The model under review builds one solid part; all positions refer to its coordinate system, in mm. Face numbers are marked on the shaded views. A direction names the side the tool comes from. Round coordinates to 2 decimals unless told otherwise and drop trailing zeros. Write each loop counter-clockwise with the first axis right and the second up, starting at its lowest first coordinate (ties: lowest second). Pieces come first, ordered by that corner, then holes.
Item 1: Add section D-D (y = 12.5). Give the boundary of the cut face in (x, z).
Item 2: Add section C-C (x = -3). Give the boundary of the cut face in (y, z), plus the area to 3 significant figures.
Item 3: Add section A-A (z = -0.5). Give the boundary of the cut face in (x, y), plus the area to 3 significant figures.
Item 4: Clearance check with flat-ended pins moving along their axes: pin 1 Ø2 at (x, z) = (17, -1) entering from +Y; pin 2 Ø4 at (x, z) = (0, 15.5) entering from -Y; pin 3 Ø4 at (y, z) = (49, -12.5) entering from +X; pin 4 Ø0.9 at (x, z) = (16.5, -0.5) entering from -Y. State where each tip first meets the part, or that it passes through.
Item 5: To check wall thickness, follow L1, parallel to X at y = 39.5, z = -7.75; L2, parallel to Y at x = -2.5, z = -10; L3, parallel to Y at x = 9, z = 5. State the ranges of each line that lie inside material, in increasing order.
Item 6: Add section B-B (y = 38.5). Give the boundary of the cut face in (x, z).
Item 7: Machinability: for the marked faces 1, 2 and 3, which of the approach directions +Z, -Z, +X, -X, +Y, -Y give a long, thin tool a straight path to every point of the face, cutting with its end or side? Answer none if there is none.
```python
from build123d import *

# Parameters (mm, degrees)
SKETCH_1_R          = 16.5
EXTRUDE_1_DEPTH     = 46
SKETCH_2_R          = 7
EXTRUDE_2_DEPTH     = 9
SKETCH_3_W          = 3
SKETCH_3_H          = 7
EXTRUDE_3_DEPTH     = 5
SKETCH_4_W          = 6
SKETCH_4_H          = 4
CUT_EXTRUDE_1_DEPTH = 3
SKETCH_5_R          = 6
EXTRUDE_4_DEPTH     = 6.5
SKETCH_7_R          = 2.5
EXTRUDE_5_DEPTH     = 70.5
EXTRUDE_START       = -23
SKETCH_8_R          = 18.5
SKETCH_8_R_2        = 16.5
EXTRUDE_6_DEPTH     = 23
SKETCH_9_R          = 1.6
CUT_EXTRUDE_2_DEPTH = 10


with BuildPart() as part:
    # 草图1 → 凸台-拉伸1 (new body)
    with BuildSketch(Plane(origin=(0, 0, 0), x_dir=(1, 0, 0), z_dir=(0, 1, 0))):
        with Locations(Location((0, 0, 0), (0, 0, 270))):
            Circle(SKETCH_1_R)
    extrude(amount=EXTRUDE_1_DEPTH)

    # 草图2 → 凸台-拉伸2 (add)
    with BuildSketch(Plane.XZ):
        with Locations(Location((0, 0, 0), (0, 0, 90))):
            Circle(SKETCH_2_R)
    extrude(amount=EXTRUDE_2_DEPTH)

    # 草图3 → 凸台-拉伸3 (add)
    with BuildSketch(Plane.XZ):
        with Locations((16.5, 0)):
            Rectangle(SKETCH_3_W, SKETCH_3_H)
    extrude(amount=EXTRUDE_3_DEPTH)

    # 草图4 → 切除-拉伸1 (cut)
    with BuildSketch(Plane(origin=(18, 0, 0), x_dir=(0, 0, -1), z_dir=(1, 0, 0))):
        with Locations((0, -2.5)):
            Rectangle(SKETCH_4_W, SKETCH_4_H)
    extrude(amount=-CUT_EXTRUDE_1_DEPTH, mode=Mode.SUBTRACT)

    # 草图5 → 凸台-拉伸4 (add)
    with BuildSketch(Plane(origin=(0, 46, 0), x_dir=(1, 0, 0), z_dir=(0, 1, 0))):
        with Locations(Location((7, 0, 0), (0, 0, 90))):
            Circle(SKETCH_5_R)
    extrude(amount=EXTRUDE_4_DEPTH)

    # 草图7 → 凸台-拉伸5 (add)
    with BuildSketch(Plane(origin=(0, 52.5, 0), x_dir=(1, 0, 0), z_dir=(0, 1, 0))):
        with Locations(Location((7, 0, 0), (0, 0, 270))):
            Circle(SKETCH_7_R)
    extrude(amount=EXTRUDE_5_DEPTH)

    # 草图8 → 凸台-拉伸6 (add)
    with BuildSketch(Plane(origin=(0, 46, 0), x_dir=(1, 0, 0), z_dir=(0, 1, 0)).offset(EXTRUDE_START)):
        with Locations(Location((0, 0, 0), (0, 0, 270))):
            Circle(SKETCH_8_R)
        with Locations(Location((0, 0, 0), (0, 0, 12.246689727))):
            Circle(SKETCH_8_R_2, mode=Mode.SUBTRACT)
    extrude(amount=EXTRUDE_6_DEPTH)

    # 草图9 → 切除-拉伸2 (cut)
    with BuildSketch(Plane(origin=(0, 46, 0), x_dir=(1, 0, 0), z_dir=(0, 1, 0))):
        with Locations(Location((-13.423393759, 7.75, 0), (0, 0, 270))):
            Circle(SKETCH_9_R)
        with Locations(Location((0, 15.5, 0), (0, 0, 270))):
            Circle(SKETCH_9_R)
        with Locations(Location((13.423393759, 7.75, 0), (0, 0, 270))):
            Circle(SKETCH_9_R)
        with Locations(Location((13.423393759, -7.75, 0), (0, 0, 270))):
            Circle(SKETCH_9_R)
        with Locations(Location((0, -15.5, 0), (0, 0, 270))):
            Circle(SKETCH_9_R)
        with Locations(Location((-13.423393759, -7.75, 0), (0, 0, 270))):
            Circle(SKETCH_9_R)
    extrude(amount=-CUT_EXTRUDE_2_DEPTH, mode=Mode.SUBTRACT)


solid = part.part
```
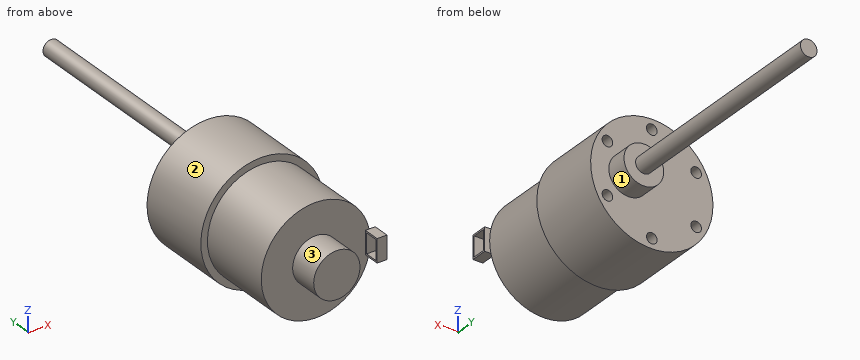
Numbers:
1. outline: circle Ø33 at (0, 0)
2. outline: (-9, -6.32) - (0, -6.32) - (0, -16.22) - (23, -16.22) - (23, -18.26) - (46, -18.26) - (46, 18.26) - (23, 18.26) - (23, 16.22) - (0, 16.22) - (0, 6.32) - (-9, 6.32) - close
2. area: 1,700 mm2
3. outline: (-18.49, 23) - (-16.49, 23) - (-16.49, 0) - (-6.98, 0) - (-6.98, -9) - (6.98, -9) - (6.98, 0) - (15, 0) - (15, -0.5) - (18, -0.5) - (18, 0) - (16.49, 0) - (16.49, 23) - (18.49, 23) - (18.49, 46) - (12.98, 46) - (12.98, 52.5) - (9.45, 52.5) - (9.45, 123) - (4.55, 123) - (4.55, 52.5) - (1.02, 52.5) - (1.02, 46) - (-18.49, 46) - close; (15, -5) - (18, -5) - (18, -4.5) - (15, -4.5) - close
3. area: 2,160 mm2
4. pin 1: stops at y = 46
4. pin 2: stops at y = 0
4. pin 3: passes through
4. pin 4: stops at y = -5
5. L1: x = -16.8 to -15.02, -11.82 to 11.82, 15.02 to 16.8
5. L2: y = 0 to 46
5. L3: y = 0 to 52.5
6. outline: circle Ø37 at (0, 0); hole circle Ø3.2 at (-13.42, -7.75); hole circle Ø3.2 at (-13.42, 7.75); hole circle Ø3.2 at (0, -15.5); hole circle Ø3.2 at (0, 15.5); hole circle Ø3.2 at (13.42, -7.75); hole circle Ø3.2 at (13.42, 7.75)
7. face 1: +Y
7. face 2: +Y, -Y
7. face 3: -Y
